```python
from build123d import *

# Parameters (mm, degrees)
PAD_DEPTH       = 3.2
SKETCH001_W     = 1
SKETCH001_H     = 22
POCKET_DEPTH    = 0.8
SKETCH002_R     = 0.5
POCKET001_DEPTH = 3.201
SKETCH003_W     = 1
SKETCH003_H     = 22
POCKET002_DEPTH = 0.8


with BuildPart() as part:
    # Sketch → Pad (new body)
    with BuildSketch(Plane.XY):
        with BuildLine():
            ThreePointArc((-2.5, 9.424038), (0, -9.75), (2.5, 9.424038))
            Line((-2.5, 9.424038), (2.5, 9.424038))
        make_face()
    extrude(amount=PAD_DEPTH)

    # Sketch001 (on Face4 of Pad) → Pocket (cut)
    with BuildSketch(Plane.XY.offset(3.2)):
        Rectangle(SKETCH001_W, SKETCH001_H)
    extrude(amount=-POCKET_DEPTH, mode=Mode.SUBTRACT)

    # Sketch002 → Pocket001 (cut, through all)
    with BuildSketch(Plane.XY):
        with Locations((0, 6)):
            Circle(SKETCH002_R)
        with Locations((0, 3)):
            Circle(SKETCH002_R)
        Circle(SKETCH002_R)
        with Locations((0, -3)):
            Circle(SKETCH002_R)
    extrude(amount=POCKET001_DEPTH, mode=Mode.SUBTRACT)

    # Sketch003 (on Face2 of Pocket001) → Pocket002 (cut)
    with BuildSketch(Plane(origin=(0, 0, 0), x_dir=(1, 0, 0), z_dir=(0, 0, -1))):
        Rectangle(SKETCH003_W, SKETCH003_H)
    extrude(amount=-POCKET002_DEPTH, mode=Mode.SUBTRACT)


solid = part.part
```
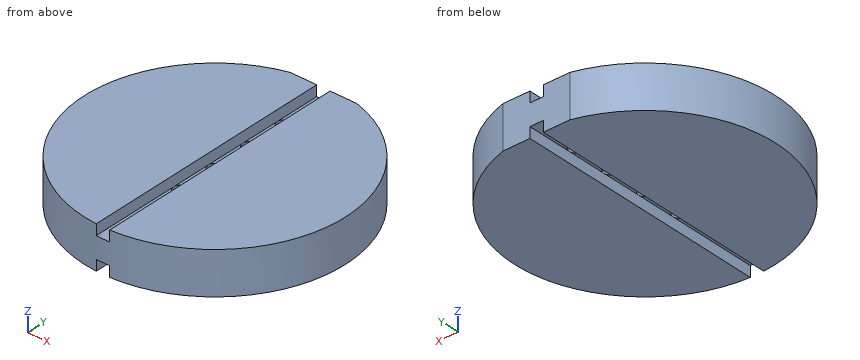
For this review, take the finished solid that the model builds, in its own axes (mm). Round coordinates to 2 decimals unless told otherwise and drop trailing zeros. Write each loop counter-clockwise with the first axis right and the second up, starting at its lowest first coordinate (ties: lowest second). Pieces come first, ordered by that corner, then holes.
1) Take a section at D-D on z = 1.3. Give the boundary of the cut face in (x, y).
Answer below:
outline: (-2.5, 9.42) arc R9.75 ccw (long way) to (2.5, 9.42) - close; hole circle Ø1 at (0, -3); hole circle Ø1 at (0, 0); hole circle Ø1 at (0, 3); hole circle Ø1 at (0, 6)
2) Take a section at C-C on y = 1.25. Give the boundary of the cut face in (x, z).
Answer below:
outline: (-9.67, 0) - (-0.5, 0) - (-0.5, 0.8) - (0.5, 0.8) - (0.5, 0) - (9.67, 0) - (9.67, 3.2) - (0.5, 3.2) - (0.5, 2.4) - (-0.5, 2.4) - (-0.5, 3.2) - (-9.67, 3.2) - close
3) Take a section at B-B on z = 2.65. Give the boundary of the cut face in (x, y).
Answer below:
outline: (-2.5, 9.42) arc R9.75 ccw to (-0.5, -9.74) - (-0.5, 9.42) - close; (0.5, -9.74) arc R9.75 ccw to (2.5, 9.42) - (0.5, 9.42) - close
4) For line 1 along X through (y, z) = (0, 1.8); line 2 along X through (y, z) = (3, 1.5); line 3 along Z through (x, y) = (0, -1), list the stretches that pass through material, from the lowest coordinate up.
Answer below:
line 1: x = -9.75 to -0.5, 0.5 to 9.75
line 2: x = -9.28 to -0.5, 0.5 to 9.28
line 3: z = 0.8 to 2.4
5) Take a section at A-A on x = 0. Give the boundary of the cut face in (y, z).
Answer below:
outline: (-9.75, 0.8) - (-3.5, 0.8) - (-3.5, 2.4) - (-9.75, 2.4) - close; (-2.5, 0.8) - (-0.5, 0.8) - (-0.5, 2.4) - (-2.5, 2.4) - close; (0.5, 0.8) - (2.5, 0.8) - (2.5, 2.4) - (0.5, 2.4) - close; (3.5, 0.8) - (5.5, 0.8) - (5.5, 2.4) - (3.5, 2.4) - close; (6.5, 0.8) - (9.42, 0.8) - (9.42, 2.4) - (6.5, 2.4) - close
6) Insertion check: pin 1 Ø0.8 at (x, y) = (0, 4) entering from -Z; pin 2 Ø0.5 at (x, y) = (0, 5) entering from +Z; pin 3 Ø1.5 at (y, z) = (2, 0.5) entering from -X. Each pin has a flat end and moves straight along its axis. Give the tip position at first contact, or say it passes through.
Answer below:
pin 1: stops at z = 0.8
pin 2: stops at z = 2.4
pin 3: stops at x = -9.67
